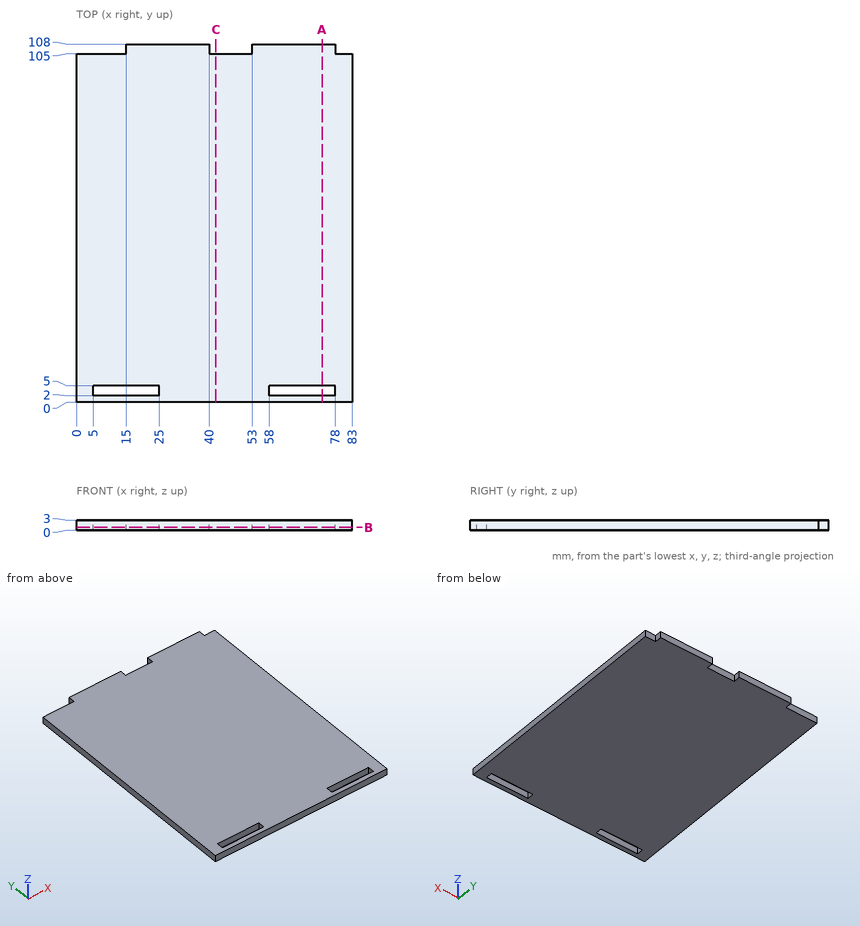
Input: dimensioned drawing with shaded views. Units: mm. Origin: part minimum x, y, z. Round coordinates to 2 decimals unless told otherwise and drop trailing zeros. Order: outer loops, then holes, each group sorted by start corner. A loop starts at its lowest first (then second) coordinate and runs counter-clockwise, first axis right, second up.
Q1. Material intervals for probe 1 along Y at (x, z) = (19, 2); probe 2 along Y at (x, z) = (8.5, 0.95); probe 3 along Y at (x, z) = (4, 2.65), sorted ascending.
Result sheet:
probe 1: y = 0 to 2, 5 to 108
probe 2: y = 0 to 2, 5 to 105
probe 3: y = 0 to 105
Q2. Section A-A, the plane x = 74. Output: boundary loops of the cut face in (y, z), and give its area (3 significant figures).
Result sheet:
outline: (0, 0) - (2, 0) - (2, 3) - (0, 3) - close; (5, 0) - (108, 0) - (108, 3) - (5, 3) - close
area: 315 mm2
Q3. Section C-C, the plane x = 42. Output: boundary loops of the cut face in (y, z).
Result sheet:
outline: (0, 0) - (105, 0) - (105, 3) - (0, 3) - close
Q4. Section B-B, the plane z = 0.95. Output: boundary loops of the cut face in (x, y).
Result sheet:
outline: (0, 0) - (83, 0) - (83, 105) - (78, 105) - (78, 108) - (53, 108) - (53, 105) - (40, 105) - (40, 108) - (15, 108) - (15, 105) - (0, 105) - close; hole (5, 2) - (25, 2) - (25, 5) - (5, 5) - close; hole (58, 2) - (78, 2) - (78, 5) - (58, 5) - close
Q5. Pin query (flat end, axial travel): pin 1 (1.5 mm diameter, centred on x = 10.5, z = 1, fed in from +Y); pin 2 (0.9 mm diameter, centred on y = 106.5, z = 2, fed in from +X); pin 3 (0.9 mm diameter, centred on y = 107, z = 1, fed in from -X). Return the tip coordinate at first contact, or that it passes through.
Result sheet:
pin 1: stops at y = 105
pin 2: stops at x = 78
pin 3: stops at x = 15
